Geometry check sheet. Reference: the model listing, model coordinates, mm. Face numbers are marked on the shaded views. A direction names the side the tool comes from. Coordinates: 2 decimals unless noted, no trailing zeros. Loops run counter-clockwise (first coordinate to the right, second up) from the corner with the lowest first, then second, coordinate; pieces in that order, holes last. Notation, with made-up numbers: M 66,41.25 L 74,41.25 A35 ccw 74,75.25 Z; hole C 24,70.25 d9. An arc over 180 degrees is marked long. Use CSV: the item, a comma, the result in double quotes.
```python
from build123d import *

# Parameters (mm, degrees)
SKETCH1_W           = 91.44
SKETCH1_H           = 68.58
BOSS_EXTRUDE1_DEPTH = 22.86
SHELL1_T            = -5.08
SKETCH2_R           = 1.397
CUT_EXTRUDE1_DEPTH  = 8.0645
FILLET1_R           = 2.54
SKETCH3_R           = 6
CUT_EXTRUDE2_DEPTH  = 5.08
SKETCH4_W           = 50.8
SKETCH4_H           = 15.875
BOSS_EXTRUDE2_DEPTH = 20.32
SKETCH5_R           = 12.9921
CUT_EXTRUDE3_DEPTH  = 104.281242035
SKETCH6_R           = 1.27
CUT_EXTRUDE4_DEPTH  = 12.6238
FILLET2_R           = 2.54


with BuildPart() as part:
    # Sketch1 → Boss-Extrude1 (new body)
    with BuildSketch(Plane.XY):
        with Locations((45.72, -34.29)):
            Rectangle(SKETCH1_W, SKETCH1_H)
    extrude(amount=BOSS_EXTRUDE1_DEPTH)

    # Shell1
    shell1_openings = [part.faces().sort_by_distance(p)[0] for p in [
        (45.72, -34.29, 22.86),
    ]]
    offset(amount=SHELL1_T, openings=shell1_openings, kind=Kind.INTERSECTION)

    # Sketch2 → Cut-Extrude1 (cut)
    with BuildSketch(Plane.XY.offset(22.86)):
        with Locations((2.794, -2.794)):
            Circle(SKETCH2_R)
        with Locations((88.646, -2.794)):
            Circle(SKETCH2_R)
        with Locations((88.646, -65.786)):
            Circle(SKETCH2_R)
        with Locations((2.794, -65.786)):
            Circle(SKETCH2_R)
    extrude(amount=-CUT_EXTRUDE1_DEPTH, mode=Mode.SUBTRACT)

    # Fillet1
    fillet1_edges = [part.edges().sort_by_distance(p)[0] for p in [
        (0, 0, 11.43),
        (91.44, 0, 11.43),
        (91.44, -68.58, 11.43),
        (0, -68.58, 11.43),
    ]]
    fillet(fillet1_edges, radius=FILLET1_R)

    # Sketch3 → Cut-Extrude2 (cut)
    with BuildSketch(Plane(origin=(0, -68.58, 0), x_dir=(-1, 0, 0), z_dir=(0, -1, 0))):
        with Locations(Location((-49.53, -11.43, 0), (0, 0, 90))):
            Circle(SKETCH3_R)
    extrude(amount=-CUT_EXTRUDE2_DEPTH, mode=Mode.SUBTRACT)

    # Sketch4 → Boss-Extrude2 (add)
    with BuildSketch(Plane(origin=(0, 0, 0), x_dir=(-1, 0, 0), z_dir=(0, 0, -1))):
        with Locations((-45.72, -34.29)):
            Rectangle(SKETCH4_W, SKETCH4_H)
    extrude(amount=BOSS_EXTRUDE2_DEPTH)

    # Sketch5 → Cut-Extrude3 (cut, through all)
    with BuildSketch(Plane.XZ.offset(42.2275)):
        with Locations((45.72, -20.32)):
            Circle(SKETCH5_R)
    extrude(amount=-CUT_EXTRUDE3_DEPTH, mode=Mode.SUBTRACT)

    # Sketch6 → Cut-Extrude4 (cut)
    with BuildSketch(Plane(origin=(0, 0, -20.32), x_dir=(-1, 0, 0), z_dir=(0, 0, -1))):
        with Locations((-26.5176, -34.29)):
            Circle(SKETCH6_R)
        with Locations((-64.9097, -34.29)):
            Circle(SKETCH6_R)
    extrude(amount=-CUT_EXTRUDE4_DEPTH, mode=Mode.SUBTRACT)

    # Fillet2
    fillet2_edges = [part.edges().sort_by_distance(p)[0] for p in [
        (20.32, -34.29, 0),
        (45.72, -26.3525, 0),
        (71.12, -34.29, 0),
        (45.72, -42.2275, 0),
    ]]
    fillet(fillet2_edges, radius=FILLET2_R)


solid = part.part
```
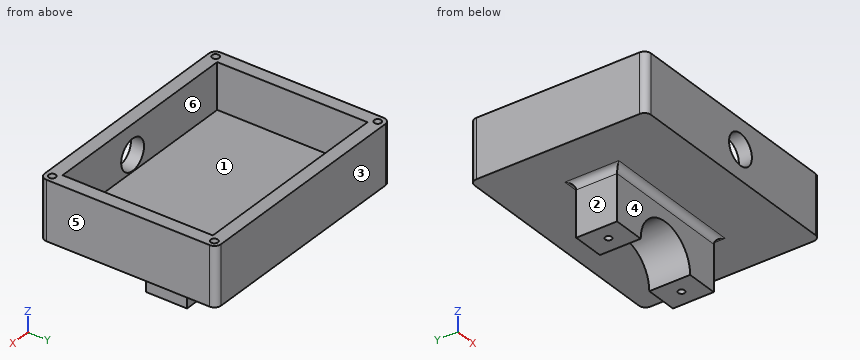
1. Thickness scan on line 1 (Y direction, x = 81.5, z = 9); line 2 (Z direction, x = 38, y = -63); line 3 (Z direction, x = 49, y = -67). Record the ranges inside material, lowest first. Write a range as [from, to].
The answers:
line 1,"[-68.58, -63.5], [-5.08, 0]"
line 2,"[0, 5.08]"
line 3,"[0, 5.45], [17.41, 22.86]"
2. Section check C-C, the plane y = -34.29. Record the cut outline in (x, z).
The answers:
outline,"M 0,0 L 17.78,0 A2.54 cw 20.32,-2.54 L 20.32,-20.32 L 25.25,-20.32 L 25.25,-7.7 L 27.79,-7.7 L 27.79,-20.32 L 32.73,-20.32 A12.99 cw 58.71,-20.32 L 63.64,-20.32 L 63.64,-7.7 L 66.18,-7.7 L 66.18,-20.32 L 71.12,-20.32 L 71.12,-2.54 A2.54 cw 73.66,0 L 91.44,0 L 91.44,22.86 L 86.36,22.86 L 86.36,5.08 L 5.08,5.08 L 5.08,22.86 L 0,22.86 Z"
3. Set-up check for the marked faces 5 and 6: record each of +Z, -Z, +X, -X, +Y, -Y from which the full face is reachable in a straight line by a thin tool's end or side.
The answers:
face 5,"+Z, -Z, +X, +Y, -Y"
face 6,"+Z"
4. Section check A-A, the plane z = 11.43. Record the cut outline in (x, y).
The answers:
outline,"M 0,-66.04 A2.54 ccw 2.54,-68.58 L 43.53,-68.58 L 43.53,-63.5 L 5.08,-63.5 L 5.08,-5.08 L 86.36,-5.08 L 86.36,-63.5 L 55.53,-63.5 L 55.53,-68.58 L 88.9,-68.58 A2.54 ccw 91.44,-66.04 L 91.44,-2.54 A2.54 ccw 88.9,0 L 2.54,0 A2.54 ccw 0,-2.54 Z"
5. Gauge pin test, flat ends, axial feed: P1, Ø3, axis at x = 48.5, y = -24, coming from the +Z side; P2, Ø12, axis at y = -41, z = -14.5, coming from the +X side; P3, Ø0.8, axis at x = 88.5, y = -2, coming from the +Z side; P4, Ø3, axis at x = 88, y = -66.5, coming from the +Z side. Record the tip position at first contact, or that the pin passes through.
The answers:
P1,"z = 5.08"
P2,"x = 71.12"
P3,"z = 14.8"
P4,"z = 22.86"
6. Release check for a two-part mould opening along Y. For the marked faces 1, 2, 3 and 4 record: +Y half, -Y half, draft (parallel to the pull), parting line (faces both ways), or undercut.
The answers:
face 1,"undercut"
face 2,"draft"
face 3,"+Y half"
face 4,"-Y half"
7. Section check B-B, the plane x = 14. Record the cut outline in (y, z), plus the area to 3 significant figures.
The answers:
outline,"M -68.58,0 L 0,0 L 0,22.86 L -5.08,22.86 L -5.08,5.08 L -63.5,5.08 L -63.5,22.86 L -68.58,22.86 Z"
area,"529 mm^2"
8. Section check D-D, the plane x = 49.53. Record the cut outline in (y, z).
The answers:
outline,"M -68.58,0 L -44.77,0 A2.54 cw -42.23,-2.54 L -42.23,-7.9 L -26.35,-7.9 L -26.35,-2.54 A2.54 cw -23.81,0 L 0,0 L 0,22.86 L -5.08,22.86 L -5.08,5.08 L -63.5,5.08 L -63.5,5.43 L -68.58,5.43 Z; M -68.58,17.43 L -63.5,17.43 L -63.5,22.86 L -68.58,22.86 Z"
